from build123d import *

# Parameters (mm, degrees)
SKETCH1_W              = 0.7874
SKETCH1_H              = 25.4
MCMASTER_2636T21_DEPTH = 28.575
CHAMFER1_SIZE          = 9.525


with BuildPart() as part:
    # Sketch1 → McMaster 2636T21 (new body, symmetric)
    with BuildSketch(Plane.XY):
        Rectangle(SKETCH1_W, SKETCH1_H)
    extrude(amount=MCMASTER_2636T21_DEPTH, both=True)

    # Chamfer1
    chamfer1_edges = [part.edges().sort_by_distance(p)[0] for p in [
        (0, -12.7, 28.575),
        (0, -12.7, -28.575),
        (0, 12.7, -28.575),
        (0, 12.7, 28.575),
    ]]
    chamfer(chamfer1_edges, length=CHAMFER1_SIZE)


solid = part.part
Here's how the part is built. I have some questions about the finished solid (model axes, mm). Coordinates: 2 decimals unless noted, no trailing zeros. Write each loop counter-clockwise with the first axis right and the second up, starting at its lowest first coordinate (ties: lowest second). Pieces come first, ordered by that corner, then holes.
1) If we section it at B-B (y = 7.75): List the corners of the cut face in (x, z) for me, plus the area to 3 significant figures.
Filled in:
outline: (-0.39, -24) - (0.39, -24) - (0.39, 24) - (-0.39, 24) - close
area: 37.8 mm2
2) If I drill on line 1 (Y direction, x = -0.1, z = -19.5); line 2 (Y direction, x = 0.2, z = -20.5); line 3 (Z direction, x = -0.15, y = -4.25), over which ranges is the centre line in solid material (lowest first)?
Filled in:
line 1: y = -12.25 to 12.25
line 2: y = -11.25 to 11.25
line 3: z = -27.5 to 27.5
3) If we section it at A-A (x = -0.1): List the corners of the cut face in (y, z) for me (3 decimals), plus the area to 3 significant figures.
Filled in:
outline: (-12.7, -19.05) - (-3.175, -28.575) - (3.175, -28.575) - (12.7, -19.05) - (12.7, 19.05) - (3.175, 28.575) - (-3.175, 28.575) - (-12.7, 19.05) - close
area: 1,270 mm2
4) If we section it at C-C (z = 21.5): List the corners of the cut face in (x, y) for me, plus the area to 3 significant figures.
Filled in:
outline: (-0.39, -10.25) - (0.39, -10.25) - (0.39, 10.25) - (-0.39, 10.25) - close
area: 16.1 mm2
